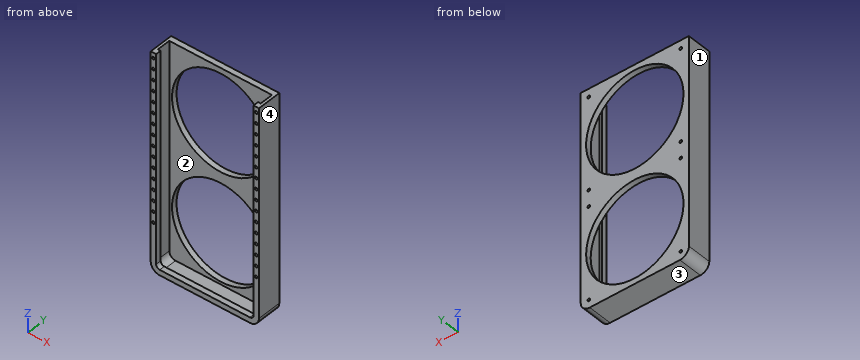
Autodesk Inventor part; units mm, degrees
ref_plane "YZ Plane" through (0, 0, 0) normal (1, 0, 0) x (0, 1, 0)
ref_plane "XZ Plane" through (0, 0, 0) normal (0, 1, 0) x (-1, 0, 0)
ref_plane "XY Plane" through (0, 0, 0) normal (0, 0, 1) x (1, 0, 0)
sketch "Sketch1" plane through (0, 0, 0) normal (0, 1, 0) x (-1, 0, 0)
  line L0 (-60, 120) -> (60, 120)
  line L1 (60, 120) -> (60, -110)
  line L2 (50, -120) -> (-50, -120)
  line L3 (-60, -110) -> (-60, 120)
  line L4 (-60, 120) -> (60, -120) construction
  line L5 (60, 120) -> (-60, -120) construction
  line L6 (-60, 120) -> (60, 120)
  line L7 (60, 120) -> (60, 0)
  line L8 (60, 0) -> (-60, 0)
  line L9 (-60, 0) -> (-60, 120)
  line L10 (60, 0) -> (-60, 120) construction
  line L11 (-60, 0) -> (60, 120) construction
  circle A0 centre (0, 60) radius 54
  line L12 (54, 60) -> (60, 60) construction
  arc A1 (50, -120) -> (60, -110) centre (50, -110) ccw
  arc A2 (-60, -110) -> (-50, -120) centre (-50, -110) ccw
  point P0 (0, 0)
  dimension "d0" = 120
  dimension "d1" = 240
  dimension "d2" = 120
  dimension "d3" = 6
  dimension "d4" = 10
extrude "Extrusion1" add sketch "Sketch1" along normal blind 6
sketch "Sketch2" plane through (0, 0, 0) normal (0, -1, 0) x (1, 0, 0)
  circle A0 centre (0, 60) radius 54 construction
  line L0 (60, 120) -> (60, -110)
  line L1 (-60, 120) -> (60, 120)
  line L2 (-60, -110) -> (-60, 120)
  arc A1 (-60, -110) -> (-50, -120) centre (-50, -110) ccw
  line L3 (50, -120) -> (-50, -120)
  arc A2 (50, -120) -> (60, -110) centre (50, -110) ccw
  line L4 (57, -110) -> (57, 117)
  line L5 (57, 117) -> (-57, 117)
  line L6 (-57, 117) -> (-57, -110)
  arc A3 (-57, -110) -> (-50, -117) centre (-50, -110) ccw
  line L7 (-50, -117) -> (50, -117)
  arc A4 (50, -117) -> (57, -110) centre (50, -110) ccw
  line L8 (57, 117) -> (57, 120)
  line L9 (-57, 117) -> (-57, 120)
  point P0 (0, 0)
  dimension "d7" = 3
extrude "Extrusion2" add sketch "Sketch2" along normal blind 15 contours L0 A2 L3 A1 L2 L1 L9 L6 A3 L7 A4 L4 L8
sketch "Sketch3" plane through (0, -15, 0) normal (0, -1, 0) x (1, 0, 0)
  line L0 (60, -110) -> (60, 120)
  line L1 (60, 120) -> (57, 120)
  line L2 (57, 120) -> (57, -110)
  arc A0 (50, -117) -> (57, -110) centre (50, -110) ccw
  line L3 (50, -117) -> (-50, -117)
  arc A1 (-57, -110) -> (-50, -117) centre (-50, -110) ccw
  line L4 (-57, -110) -> (-57, 120)
  line L5 (-57, 120) -> (-60, 120)
  line L6 (-60, 120) -> (-60, -110)
  arc A2 (-60, -110) -> (-50, -120) centre (-50, -110) ccw
  line L7 (-50, -120) -> (50, -120)
  arc A3 (50, -120) -> (60, -110) centre (50, -110) ccw
  line L8 (57, 120) -> (54, 120)
  line L9 (-60, 120) -> (60, 120) construction
  line L10 (54, 120) -> (54, -110)
  line L11 (50, -114) -> (25, -114)
  arc A4 (50, -114) -> (54, -110) centre (50, -110) ccw
  line L12 (0, 0) -> (0, -136) construction
  line L13 (-57, 120) -> (-54, 120)
  line L14 (-54, 120) -> (-54, -110)
  line L15 (-50, -114) -> (25, -114)
  arc A5 (-54, -110) -> (-50, -114) centre (-50, -110) ccw
  dimension "d10" = 3
extrude "Extrusion3" add sketch "Sketch3" along normal blind 6
sketch "Sketch5" plane through (0, 6, 0) normal (0, 1, 0) x (1, 0, 0)
  circle A0 centre (0, -60) radius 54
  line L0 (60, -120) -> (60, 110)
  arc A1 (60, 110) -> (50, 120) centre (50, 110) ccw
  line L1 (50, 120) -> (-50, 120)
  arc A2 (-50, 120) -> (-60, 110) centre (-50, 110) ccw
  line L2 (-60, 110) -> (-60, -120)
  line L3 (-60, -120) -> (60, -120)
  line L4 (-67.6504, 0) -> (67.3496, 0) construction
  circle A3 centre (0, 60) radius 54
  point P0 (0, 0)
extrude "Extrusion4" cut sketch "Sketch5" against normal up to next contours A3
sketch "Sketch6" plane through (0, 6, 0) normal (0, 1, 0) x (1, 0, 0)
  circle A0 centre (0, -60) radius 54
  circle A1 centre (0, 60) radius 54
  circle A2 centre (0, 60) radius 54
  circle A3 centre (0, -60) radius 54
  line L0 (60, -120) -> (60, 110)
  arc A4 (60, 110) -> (50, 120) centre (50, 110) ccw
  line L1 (50, 120) -> (-50, 120)
  arc A5 (-50, 120) -> (-60, 110) centre (-50, 110) ccw
  line L2 (-60, 110) -> (-60, -120)
  line L3 (-60, -120) -> (60, -120)
  line L4 (-50.0326, 0) -> (43.9674, 0) construction
  line L5 (0, -60) -> (-70, -60) construction
  line L6 (0, -60) -> (0, -118) construction
  point P0 (0, 0)
  point P1 (-51, -9)
  point P2 (-51, -111)
  point P3 (51, -9)
  point P4 (51, -111)
  point P5 (-51, 9)
  point P6 (-51, 111)
  point P7 (51, 111)
  point P8 (51, 9)
  dimension "d15" = 18
  dimension "d16" = 9
hole "Hole1" at (-51, 6, 9) at (-51, 6, 111) at (51, 6, 111) at (51, 6, 9) at (-51, 6, -111) at (-51, 6, -9) at (51, 6, -111) at (51, 6, -9) direction (0, -1, 0) diameter 3 depth 4 tip angle 118
sketch "Sketch7" plane through (0, -21, 0) normal (0, -1, 0) x (1, 0, 0)
  line L0 (57, 120) -> (57, -110) construction
  line L1 (57, -110) -> (57, 120)
  line L2 (-57, -110) -> (-57, 120) construction
  line L3 (-57, 120) -> (-57, -110)
  line L4 (57, 120) -> (57, -110)
  line L5 (0, 119) -> (0, 0) construction
  point P0 (57, 60)
  point P1 (57, -60)
  point P2 (57, 114)
  point P3 (-57, 114)
  point P4 (-57, 102)
  point P5 (57, 102)
  point P6 (-57, 90)
  point P7 (57, 90)
  point P8 (-57, 78)
  point P9 (57, 78)
  point P10 (-57, 66)
  point P11 (57, 66)
  point P12 (-57, 54)
  point P13 (57, 54)
  point P14 (-57, 42)
  point P15 (57, 42)
  point P16 (-57, 30)
  point P17 (57, 30)
  point P18 (-57, 18)
  point P19 (57, 18)
  point P20 (-57, 6)
  point P21 (57, 6)
  point P22 (-57, -6)
  point P23 (57, -6)
  point P24 (-57, -18)
  point P25 (57, -18)
  point P26 (-57, -30)
  point P27 (57, -30)
  point P28 (-57, -42)
  point P29 (57, -42)
  point P30 (-57, -54)
  point P31 (57, -54)
  point P32 (-57, -66)
  point P33 (57, -66)
  dimension "d24" = 6
  dimension "d27" = 12
hole "Hole2" at (57, -21, 114) at (-57, -21, 114) at (-57, -21, 102) at (57, -21, 102) at (-57, -21, 90) at (57, -21, 90) at (-57, -21, 78) at (57, -21, 78) at (-57, -21, 66) at (57, -21, 66) at (-57, -21, 54) at (57, -21, 54) at (-57, -21, 42) at (57, -21, 42) at (-57, -21, 30) at (57, -21, 30) at (-57, -21, 18) at (57, -21, 18) at (-57, -21, 6) at (57, -21, 6) at (-57, -21, -6) at (57, -21, -6) at (-57, -21, -18) at (57, -21, -18) at (-57, -21, -30) at (57, -21, -30) at (-57, -21, -42) at (57, -21, -42) at (-57, -21, -54) at (57, -21, -54) at (-57, -21, -66) at (57, -21, -66) direction (0, 1, 0) diameter 3 depth 4 tip angle 118
equation "\"d0\" = hull_width"
equation "\"d1\" = hull_length"
equation "\"d2\" = hull_width"
equation "\"d3\" = 2 * thickness"
equation "\"d4\" = roundness"
equation "\"d5\" = 2 * thickness"
equation "\"d7\" = thickness"
equation "\"d8\" = 5 * thickness"
equation "\"d10\" = thickness"
equation "\"d11\" = 2 * thickness"
equation "\"d13\" = 2 * thickness"
equation "\"d22\" = 1.33333 * thickness"
equation "\"d37\" = 1.33333 * thickness"
equation "\"thickness\" = 3"
equation "\"roundness\" = 10"
equation "\"hull_width\" = 120"
equation "\"hull_length\" = 2 * hull_width"
properties part number "Cup_Dispenser_Hull"
Verification items for the finished model (mm, model axes). Face numbers are marked on the shaded views. Coordinates: 2 decimals unless noted, no trailing zeros. Order: outer loops, then holes, each group sorted by start corner. A loop starts at its lowest first (then second) coordinate and runs counter-clockwise, first axis right, second up. Notation, with made-up numbers: (36.5, 7) - (94.5, 7) arc R11 cw to (94.5, 13) - close; hole circle Ø11 at (77, 70). An arc over 180 degrees is marked (long way). Return JSON: item names as keys, results as strings.
(1) Section check D-D, the plane x = -42.5. Record the cut outline in (y, z), and give its area (3 significant figures).
Filled sheet:
{"outline": "(-21, -120) - (6, -120) - (6, -93.31) - (0, -93.31) - (0, -117) - (-15, -117) - (-15, -114) - (-21, -114) - close; (0, -26.69) - (6, -26.69) - (6, 26.69) - (0, 26.69) - close; (0, 93.31) - (6, 93.31) - (6, 120) - (0, 120) - close", "area": "721 mm^2"}
(2) Section check A-A, the plane z = -60. Record the cut outline in (x, y), and give its area (3 significant figures).
Filled sheet:
{"outline": "(-60, -21) - (-54, -21) - (-54, -15) - (-57, -15) - (-57, 0) - (-54, 0) - (-54, 6) - (-60, 6) - close; (54, -21) - (60, -21) - (60, 6) - (54, 6) - (54, 0) - (57, 0) - (57, -15) - (54, -15) - close", "area": "234 mm^2"}
(3) Section check C-C, the plane y = -6.75. Record the cut outline in (x, z).
Filled sheet:
{"outline": "(-60, -110) arc R10 ccw to (-50, -120) - (50, -120) arc R10 ccw to (60, -110) - (60, 120) - (57, 120) - (57, -110) arc R7 cw to (50, -117) - (-50, -117) arc R7 cw to (-57, -110) - (-57, 120) - (-60, 120) - close"}
(4) Section check B-B, the plane x = 20. Record the cut outline in (y, z), and give its area (3 significant figures).
Filled sheet:
{"outline": "(-21, -120) - (6, -120) - (6, -110.16) - (0, -110.16) - (0, -117) - (-15, -117) - (-15, -114) - (-21, -114) - close; (0, -9.84) - (6, -9.84) - (6, 9.84) - (0, 9.84) - close; (0, 110.16) - (6, 110.16) - (6, 120) - (0, 120) - close", "area": "317 mm^2"}
(5) Go/stop test with flat-tipped pins: pin 1 (3.5 mm diameter, centred on x = -51, z = 9, fed in from -Y); pin 2 (10 mm diameter, centred on x = 39.5, y = -12.5, fed in from +Z). Record where each tip stops, or that it passes through.
Filled sheet:
{"pin 1": "stops at y = 0", "pin 2": "stops at z = -114"}
(6) Mould release check, pull along X, two halves, no side actions. Record for the marked faces 1, 2, 3 and 4: pulls with the +X half, pulls with the -X half, needs draft (parallel to the pull), parting line crosses it, or undercut.
Filled sheet:
{"face 1": "pulls with the -X half", "face 2": "undercut", "face 3": "needs draft", "face 4": "pulls with the +X half"}
(7) Thickness scan on line 1 along X through (y, z) = (-20.15, -18); line 2 along X through (y, z) = (-2.5, 5.5); line 3 along X through (y, z) = (3.15, -60). Record the ranges inside material, lowest first.
Filled sheet:
{"line 1": "x = -60 to -58.5, -55.5 to -54, 54 to 55.5, 58.5 to 60", "line 2": "x = -60 to -57, 57 to 60", "line 3": "x = -60 to -54, 54 to 60"}
